Build history of the part. All positions in model axes, mm. Give positions to 0.01 mm unless a question says otherwise; leave off trailing zeros. Write each loop counter-clockwise with the first axis right and the second up, starting at its lowest first coordinate (ties: lowest second). Pieces come first, ordered by that corner, then holes.
from build123d import *

# Parameters (mm, degrees)
SKETCH1_R           = 1.5
BOSS_EXTRUDE1_DEPTH = 2.325
CHAMFER1_SIZE       = 0.125
FILLET1_R           = 0.25


with BuildPart() as part:
    # Sketch1 → Boss-Extrude1 (new body)
    with BuildSketch(Plane(origin=(0, 0, 0), x_dir=(1, 0, 0), z_dir=(0, 1, 0))):
        Polygon((3.117691454, 0), (1.558845727, 2.7), (-1.558845727, 2.7), (-3.117691454, 0), (-1.558845727, -2.7), (1.558845727, -2.7), align=None)
        with Locations(Location((0, 0, 0), (0, 0, 270))):
            Circle(SKETCH1_R, mode=Mode.SUBTRACT)
    extrude(amount=BOSS_EXTRUDE1_DEPTH)

    # Chamfer1
    chamfer1_edges = [part.edges().sort_by_distance(p)[0] for p in [
        (0, 2.325, -2.7),
        (-2.33826859, 2.325, -1.35),
        (-2.33826859, 2.325, 1.35),
        (0, 2.325, 2.7),
        (2.33826859, 2.325, 1.35),
        (0, 0, 2.7),
        (-2.33826859, 0, 1.35),
        (-2.33826859, 0, -1.35),
        (0, 0, -2.7),
        (2.33826859, 0, -1.35),
        (2.33826859, 0, 1.35),
        (2.33826859, 2.325, -1.35),
    ]]
    chamfer(chamfer1_edges, length=CHAMFER1_SIZE)

    # Fillet1
    fillet1_edges = [part.edges().sort_by_distance(p)[0] for p in [
        (0, 0, -1.5),
        (0, 2.325, -1.5),
        (-2.230015415, 0, 1.2875),
        (0, 0, 2.575),
        (2.230015415, 0, 1.2875),
        (-2.230015415, 0, -1.2875),
        (0, 0, -2.575),
        (2.230015415, 0, -1.2875),
        (-2.230015415, 2.325, 1.2875),
        (-2.230015415, 2.325, -1.2875),
        (0, 2.325, -2.575),
        (2.230015415, 2.325, -1.2875),
        (2.230015415, 2.325, 1.2875),
        (0, 2.325, 2.575),
    ]]
    fillet(fillet1_edges, radius=FILLET1_R)


solid = part.part
(1) Saw through at A-A, the plane x = 0. List the corners of the cut face in (y, z) (3 decimals).
(2) Probe line 1 (X direction, y = 1.8, z = 0.45); line 2 (Z direction, x = 0.25, y = 1.2); line 3 (X direction, y = 0.6, z = 1.05). List the from-to ranges inside material, lowest first.
(3) Saw through at B-B, the plane y = 0.5. List the corners of the cut face in (x, z).
(4) Drop a flat-ended pin along its axis: pin 1 (2.5 mm diameter, centred on x = 0, z = 0, fed in from -Y). Give the stop position or say it passes through.
(5) Mould opens along Y. For faces 1 (the face through (1, 2.325, -2)), 2 (the face through (-2.327, 1.148, -1.369)) say: +Y half, -Y half, draft (parallel to the pull), parting line (faces both ways), or undercut.
Computed values:
1. outline: (0, -2.471) arc R0.25 ccw to (0.073, -2.648) - (0.125, -2.7) - (2.2, -2.7) - (2.252, -2.648) arc R0.25 ccw to (2.325, -2.471) - (2.325, -1.75) arc R0.25 ccw to (2.075, -1.5) - (0.25, -1.5) arc R0.25 ccw to (0, -1.75) - close; (0, 1.75) arc R0.25 ccw to (0.25, 1.5) - (2.075, 1.5) arc R0.25 ccw to (2.325, 1.75) - (2.325, 2.471) arc R0.25 ccw to (2.252, 2.648) - (2.2, 2.7) - (0.125, 2.7) - (0.073, 2.648) arc R0.25 ccw to (0, 2.471) - close
2. line 1: x = -2.86 to -1.43, 1.43 to 2.86
2. line 2: z = -2.7 to -1.48, 1.48 to 2.7
2. line 3: x = -2.51 to -1.07, 1.07 to 2.51
3. outline: (-3.12, 0) - (-1.56, -2.7) - (1.56, -2.7) - (3.12, 0) - (1.56, 2.7) - (-1.56, 2.7) - close; hole circle Ø3 at (0, 0)
4. pin 1: passes through
5. face 1: +Y half
5. face 2: draft
